Can you work these out from the model? Positions are in its coordinate system, mm. Face numbers are marked on the shaded views. A direction names the side the tool comes from. Round coordinates to 2 decimals unless told otherwise and drop trailing zeros. Order: outer loops, then holes, each group sorted by start corner. A loop starts at its lowest first (then second) coordinate and runs counter-clockwise, first axis right, second up. Notation, with made-up numbers: (33.5, -9.75) -> (46.5, -9.75) arc R6 cw to (46.5, -4.75) -> close; hole circle Ø1 at (63.25, -16.5). An arc over 180 degrees is marked (long way). One line per item, written item: value.
```python
from build123d import *

# Parameters (mm, degrees)
BOX002_W     = 20
BOX002_H     = 20
BOX002_DEPTH = 10
BOX001_W     = 30
BOX001_H     = 20
BOX001_DEPTH = 10
BOX_W        = 70
BOX_H        = 20
BOX_DEPTH    = 4
FILLET_R     = 2


with BuildPart() as cube002:
    # Box002 → Box002 (new body)
    with BuildSketch(Plane(origin=(35, 0, 4), x_dir=(1, 0, 0), z_dir=(0, 0, 1))):
        with Locations((10, 10)):
            Rectangle(BOX002_W, BOX002_H)
    extrude(amount=BOX002_DEPTH)


with BuildPart() as cube001:
    # Box001 → Box001 (new body)
    with BuildSketch(Plane(origin=(30, 0, 4), x_dir=(1, 0, 0), z_dir=(0, 0, 1))):
        with Locations((15, 10)):
            Rectangle(BOX001_W, BOX001_H)
    extrude(amount=BOX001_DEPTH)


with BuildPart() as fillet_body:
    # Box → Box (new body)
    with BuildSketch(Plane.XY):
        with Locations((35, 10)):
            Rectangle(BOX_W, BOX_H)
    extrude(amount=BOX_DEPTH)

    # Fusion: union Cube001
    add(cube001.part)

    # Cut: cut Cube002
    add(cube002.part, mode=Mode.SUBTRACT)

    # Fillet
    fillet_edges = [fillet_body.edges().sort_by_distance(p)[0] for p in [
        (0, 10, 4),
        (30, 10, 4),
        (70, 10, 4),
        (60, 10, 4),
        (30, 10, 14),
        (35, 10, 14),
        (55, 10, 14),
        (60, 10, 14),
    ]]
    fillet(fillet_edges, radius=FILLET_R)


solid = fillet_body.part
```
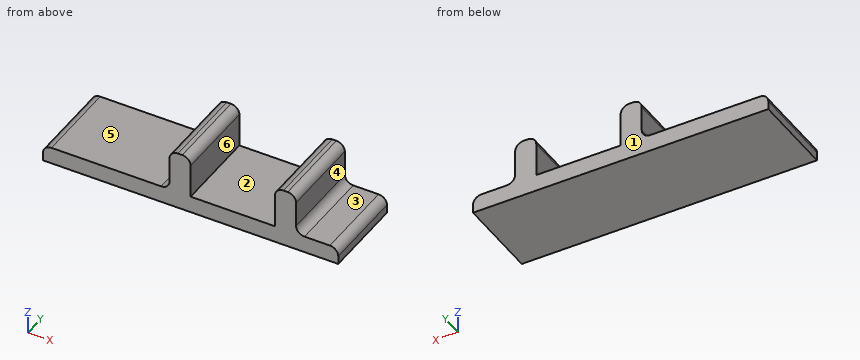
Q1. Please list where these lines run through material, in increasing order: line 1 along X through (y, z) = (18, 6.75); line 2 along Z through (x, y) = (5, 4); line 3 along X through (y, z) = (10.5, 4.25).
Answers below:
line 1: 30 to 35, 55 to 60
line 2: 0 to 4
line 3: 28.97 to 35, 55 to 61.03
Q2. Will these pins go through, and if not, where does the flat tip stop? pin 1 Ø5 at (x, y) = (66, 9) entering from +Z; pin 2 Ø6.5 at (y, z) = (12.5, 8) entering from +X; pin 3 Ø2.5 at (y, z) = (7, 7.5) entering from -X.
Answers below:
pin 1: z = 4
pin 2: x = 60.44
pin 3: x = 30
Q3. I want a section at C-C on x = 22.5. List the corners of the cut face in (y, z) for me.
Answers below:
outline: (0, 0) -> (20, 0) -> (20, 4) -> (0, 4) -> close
Q4. We'd pull the mould along X, two halves only. Please class the marked faces 4, 5 and 6: released by +X, released by -X, zero draft, split by the parting line, or undercut.
Answers below:
face 4: released by +X
face 5: zero draft
face 6: undercut
Q5. I want a section at A-A on z = 9.5. List the corners of the cut face in (x, y) for me.
Answers below:
outline: (30, 0) -> (35, 0) -> (35, 20) -> (30, 20) -> close; (55, 0) -> (60, 0) -> (60, 20) -> (55, 20) -> close
Q6. On a 3-axis mill with a long thin cutter (end or side, diameter ignored), from which of +Z, -Z, +X, -X, +Y, -Y can I reach the whole of each face in a straight line? I mean the marked faces 1, 2 and 3. Say none if no direction works.
Answers below:
face 1: +Z, -Z, +X, -X, +Y
face 2: +Z, +Y, -Y
face 3: +Z, +X, +Y, -Y
Q7. I want a section at B-B on y = 3.5. List the corners of the cut face in (x, z) for me.
Answers below:
outline: (0, 0) -> (70, 0) -> (70, 2) arc R2 ccw to (68, 4) -> (62, 4) arc R2 cw to (60, 6) -> (60, 12) arc R2 ccw to (58, 14) -> (57, 14) arc R2 ccw to (55, 12) -> (55, 4) -> (35, 4) -> (35, 12) arc R2 ccw to (33, 14) -> (32, 14) arc R2 ccw to (30, 12) -> (30, 6) arc R2 cw to (28, 4) -> (2, 4) arc R2 ccw to (0, 2) -> close
